Source: CAD feature listing. Evaluate the final solid. Frame: model axes, mm. Give positions to 0.01 mm unless a question says otherwise; leave off trailing zeros. Write each loop counter-clockwise with the first axis right and the second up, starting at its lowest first coordinate (ties: lowest second). Pieces come first, ordered by that corner, then holes.
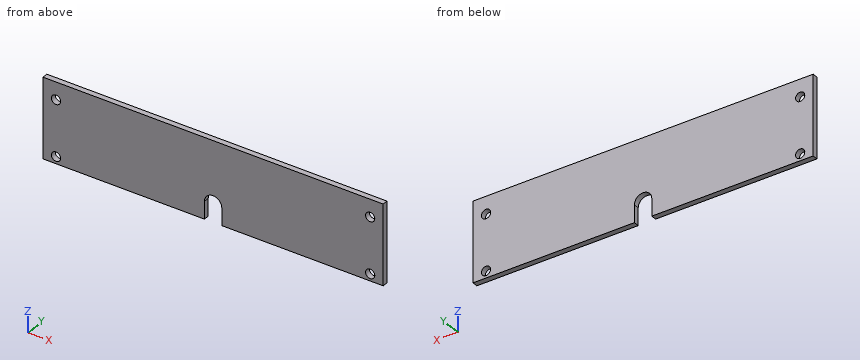
```python
from build123d import *

# Parameters (mm, degrees)
SKETCH1_W            = 196
SKETCH1_H            = 46
BOSS_EXTRUDE1_DEPTH  = 3.175
SKETCH2_W            = 10
SKETCH2_H            = 10
CUT_EXTRUDE1_DEPTH   = 3.175
M5_CLEARANCE_HOLE1_D = 5.3


with BuildPart() as part:
    # Sketch1 → Boss-Extrude1 (new body)
    with BuildSketch(Plane(origin=(0, 0, 0), x_dir=(1, 0, 0), z_dir=(0, 1, 0))):
        with Locations((98, 23)):
            Rectangle(SKETCH1_W, SKETCH1_H)
    extrude(amount=BOSS_EXTRUDE1_DEPTH)

    # Sketch2 → Cut-Extrude1 (cut)
    with BuildSketch(Plane(origin=(0, 3.175, 0), x_dir=(1, 0, 0), z_dir=(0, 1, 0))):
        with Locations((98, 41)):
            Rectangle(SKETCH2_W, SKETCH2_H)
        with BuildLine():
            ThreePointArc((93, 36), (98, 31), (103, 36))
            Line((103, 36), (93, 36))
        make_face()
    extrude(amount=-CUT_EXTRUDE1_DEPTH, mode=Mode.SUBTRACT)

    # M5 Clearance Hole1 (through all)
    with Locations(Plane(origin=(0, 3.175, 0), x_dir=(1, 0, 0), z_dir=(0, 1, 0))):
        with Locations((188.5, 10), (7.5, 10), (188.5, 42), (7.5, 42)):
            Hole(M5_CLEARANCE_HOLE1_D / 2)


solid = part.part
```
1. Cut plane D-D, the plane x = 98. Return the cut outline in (y, z) (3 decimals), then the cut area to 3 significant figures.
2. Contact query for a flat-ended pin moving along its axis: P1, Ø4, axis at x = 188.5, z = -42, coming from the +Y side. Output: stop coordinate, or through.
3. Cut plane B-B, the plane x = 7.5. Return the cut outline in (y, z) (3 decimals), then the cut area to 3 significant figures.
4. Cut plane A-A, the plane y = 1.85. Return the cut outline in (x, z), then the cut area to 3 significant figures.
5. Line query: L1, parallel to Z at x = 188.5, y = 1.2; L2, parallel to X at y = 2.5, z = -42; L3, parallel to X at y = 1, z = -10. Output: solid intervals per line, ascending.
6. Cut plane C-C, the plane z = -42. Return the cut outline in (x, y) (3 decimals), then the cut area to 3 significant figures.
Response values:
1. outline: (0, -31) - (3.175, -31) - (3.175, 0) - (0, 0) - close
1. area: 98.4 mm2
2. P1: passes through
3. outline: (0, -46) - (3.175, -46) - (3.175, -44.65) - (0, -44.65) - close; (0, -39.35) - (3.175, -39.35) - (3.175, -12.65) - (0, -12.65) - close; (0, -7.35) - (3.175, -7.35) - (3.175, 0) - (0, 0) - close
3. area: 112 mm2
4. outline: (0, -46) - (93, -46) - (93, -36) arc R5 cw to (103, -36) - (103, -46) - (196, -46) - (196, 0) - (0, 0) - close; hole circle Ø5.3 at (7.5, -42); hole circle Ø5.3 at (7.5, -10); hole circle Ø5.3 at (188.5, -42); hole circle Ø5.3 at (188.5, -10)
4. area: 8,790 mm2
5. L1: z = -46 to -44.65, -39.35 to -12.65, -7.35 to 0
5. L2: x = 0 to 4.85, 10.15 to 93, 103 to 185.85, 191.15 to 196
5. L3: x = 0 to 4.85, 10.15 to 185.85, 191.15 to 196
6. outline: (0, 0) - (4.85, 0) - (4.85, 3.175) - (0, 3.175) - close; (10.15, 0) - (93, 0) - (93, 3.175) - (10.15, 3.175) - close; (103, 0) - (185.85, 0) - (185.85, 3.175) - (103, 3.175) - close; (191.15, 0) - (196, 0) - (196, 3.175) - (191.15, 3.175) - close
6. area: 557 mm2
